The model under review builds one solid part; all positions refer to its coordinate system, in mm. A direction names the side the tool comes from. Coordinates: 2 decimals unless noted, no trailing zeros. Order: outer loops, then holes, each group sorted by start corner. A loop starts at its lowest first (then second) coordinate and runs counter-clockwise, first axis right, second up.
from build123d import *

# Parameters (mm, degrees)
SKETCH2_W                      = 17
SKETCH2_H                      = 17
BOSS_EXTRUDE1_DEPTH            = 3
SKETCH3_R                      = 2.2
CUT_EXTRUDE1_DEPTH             = 1.5
M2_CLEARANCE_HOLE1_D           = 2.4
M2_CLEARANCE_HOLE1_CSINK_D     = 2.45
M2_CLEARANCE_HOLE1_CSINK_ANGLE = 90
BOSS_EXTRUDE2_DEPTH            = 50
BOSS_EXTRUDE2_DRAFT            = 1.8
BOSS_EXTRUDE2_PROFILE_2_DEPTH  = 50
BOSS_EXTRUDE2_PROFILE_2_DRAFT  = 1.8
BOSS_EXTRUDE2_PROFILE_3_DEPTH  = 50
BOSS_EXTRUDE2_PROFILE_3_DRAFT  = 1.8
BOSS_EXTRUDE2_PROFILE_4_DEPTH  = 50
BOSS_EXTRUDE2_PROFILE_4_DRAFT  = 1.8
FILLET1_R                      = 6
FILLET2_R                      = 2
BOSS_EXTRUDE3_DEPTH            = 1.5


with BuildPart() as part:
    # Sketch2 → Boss-Extrude1 (new body)
    with BuildSketch(Plane(origin=(0, 0, 0), x_dir=(0, 1, 0), z_dir=(0, 0, 1))):
        with BuildLine():
            Line((-38.870057685, 34.627416998), (-34.627416998, 38.870057685))
            Line((-34.627416998, 38.870057685), (-14.186291501, 18.428932188))
            ThreePointArc((-14.186291501, 18.428932188), (-10.942058013, 16.261204675), (-7.115223689, 15.5))
            Line((-7.115223689, 15.5), (7.115223689, 15.5))
            ThreePointArc((7.115223689, 15.5), (10.942058013, 16.261204675), (14.186291501, 18.428932188))
            Line((14.186291501, 18.428932188), (34.627416998, 38.870057685))
            Line((34.627416998, 38.870057685), (38.870057685, 34.627416998))
            Line((38.870057685, 34.627416998), (18.428932188, 14.186291501))
            ThreePointArc((18.428932188, 14.186291501), (16.261204675, 10.942058013), (15.5, 7.115223689))
            Line((15.5, 7.115223689), (15.5, -7.115223689))
            ThreePointArc((15.5, -7.115223689), (16.261204675, -10.942058013), (18.428932188, -14.186291501))
            Line((18.428932188, -14.186291501), (38.870057685, -34.627416998))
            Line((38.870057685, -34.627416998), (34.627416998, -38.870057685))
            Line((34.627416998, -38.870057685), (14.186291501, -18.428932188))
            ThreePointArc((14.186291501, -18.428932188), (10.942058013, -16.261204675), (7.115223689, -15.5))
            Line((7.115223689, -15.5), (-7.115223689, -15.5))
            ThreePointArc((-7.115223689, -15.5), (-10.942058013, -16.261204675), (-14.186291501, -18.428932188))
            Line((-14.186291501, -18.428932188), (-34.627416998, -38.870057685))
            Line((-34.627416998, -38.870057685), (-38.870057685, -34.627416998))
            Line((-38.870057685, -34.627416998), (-18.428932188, -14.186291501))
            ThreePointArc((-18.428932188, -14.186291501), (-16.261204675, -10.942058013), (-15.5, -7.115223689))
            Line((-15.5, -7.115223689), (-15.5, 7.115223689))
            ThreePointArc((-15.5, 7.115223689), (-16.261204675, 10.942058013), (-18.428932188, 14.186291501))
            Line((-18.428932188, 14.186291501), (-38.870057685, 34.627416998))
        make_face()
        Rectangle(SKETCH2_W, SKETCH2_H, mode=Mode.SUBTRACT)
    extrude(amount=BOSS_EXTRUDE1_DEPTH)

    # Sketch3 → Cut-Extrude1 (cut)
    with BuildSketch(Plane.XY.offset(3)):
        with Locations((-12.5, 12.5)):
            Circle(SKETCH3_R)
        with Locations((12.5, 12.5)):
            Circle(SKETCH3_R)
        with Locations((12.5, -12.5)):
            Circle(SKETCH3_R)
        with Locations((-12.5, -12.5)):
            Circle(SKETCH3_R)
    extrude(amount=-CUT_EXTRUDE1_DEPTH, mode=Mode.SUBTRACT)

    # M2 Clearance Hole1 (through all)
    with Locations(Plane.XY.offset(3)):
        with Locations((12.5, 12.5), (-12.5, -12.5), (-12.5, 12.5), (12.5, -12.5)):
            CounterSinkHole(M2_CLEARANCE_HOLE1_D / 2, M2_CLEARANCE_HOLE1_CSINK_D / 2, counter_sink_angle=M2_CLEARANCE_HOLE1_CSINK_ANGLE)


with BuildPart() as boss_extrude2_tool:
    # Sketch7 → Boss-Extrude2 (with draft: the straight prism first)
    with BuildSketch(Plane(origin=(0, 0, 0), x_dir=(1, 0, 0), z_dir=(0, 0, -1))):
        Polygon((28.263455967, 31.091883092), (31.091883092, 28.263455967), (38.162950904, 35.334523779), (35.334523779, 38.162950904), align=None)
    extrude(amount=BOSS_EXTRUDE2_DEPTH)
    # Boss-Extrude2: the draft: its side faces are tilted about the plane it starts from
    boss_extrude2_sides = [boss_extrude2_tool.faces().sort_by_distance(p)[0] for p in [
        (29.67766953, -29.67766953, -25),
        (34.627416998, -31.798989873, -25),
        (36.748737342, -36.748737342, -25),
        (31.798989873, -34.627416998, -25),
    ]]
    draft(boss_extrude2_sides, Plane(origin=(0, 0, 0), x_dir=(1, 0, 0), z_dir=(0, 0, -1)), BOSS_EXTRUDE2_DRAFT)


with BuildPart() as part_1:
    add(part.part)

    # Boss-Extrude2: add boss_extrude2_tool
    add(boss_extrude2_tool.part)


with BuildPart() as boss_extrude2_profile_2_tool:
    # Sketch7 → Boss-Extrude2 profile 2 (with draft: the straight prism first)
    with BuildSketch(Plane(origin=(0, 0, 0), x_dir=(1, 0, 0), z_dir=(0, 0, -1))):
        Polygon((31.091883092, -28.263455967), (28.263455967, -31.091883092), (35.334523779, -38.162950904), (38.162950904, -35.334523779), align=None)
    extrude(amount=BOSS_EXTRUDE2_PROFILE_2_DEPTH)
    # Boss-Extrude2 profile 2: the draft: its side faces are tilted about the plane it starts from
    boss_extrude2_profile_2_sides = [boss_extrude2_profile_2_tool.faces().sort_by_distance(p)[0] for p in [
        (29.67766953, 29.67766953, -25),
        (31.798989873, 34.627416998, -25),
        (36.748737342, 36.748737342, -25),
        (34.627416998, 31.798989873, -25),
    ]]
    draft(boss_extrude2_profile_2_sides, Plane(origin=(0, 0, 0), x_dir=(1, 0, 0), z_dir=(0, 0, -1)), BOSS_EXTRUDE2_PROFILE_2_DRAFT)


with BuildPart() as part_2:
    add(part_1.part)

    # Boss-Extrude2 profile 2: add boss_extrude2_profile_2_tool
    add(boss_extrude2_profile_2_tool.part)


with BuildPart() as boss_extrude2_profile_3_tool:
    # Sketch7 → Boss-Extrude2 profile 3 (with draft: the straight prism first)
    with BuildSketch(Plane(origin=(0, 0, 0), x_dir=(1, 0, 0), z_dir=(0, 0, -1))):
        Polygon((-28.263455967, -31.091883092), (-31.091883092, -28.263455967), (-38.162950904, -35.334523779), (-35.334523779, -38.162950904), align=None)
    extrude(amount=BOSS_EXTRUDE2_PROFILE_3_DEPTH)
    # Boss-Extrude2 profile 3: the draft: its side faces are tilted about the plane it starts from
    boss_extrude2_profile_3_sides = [boss_extrude2_profile_3_tool.faces().sort_by_distance(p)[0] for p in [
        (-29.67766953, 29.67766953, -25),
        (-34.627416998, 31.798989873, -25),
        (-36.748737342, 36.748737342, -25),
        (-31.798989873, 34.627416998, -25),
    ]]
    draft(boss_extrude2_profile_3_sides, Plane(origin=(0, 0, 0), x_dir=(1, 0, 0), z_dir=(0, 0, -1)), BOSS_EXTRUDE2_PROFILE_3_DRAFT)


with BuildPart() as part_3:
    add(part_2.part)

    # Boss-Extrude2 profile 3: add boss_extrude2_profile_3_tool
    add(boss_extrude2_profile_3_tool.part)


with BuildPart() as boss_extrude2_profile_4_tool:
    # Sketch7 → Boss-Extrude2 profile 4 (with draft: the straight prism first)
    with BuildSketch(Plane(origin=(0, 0, 0), x_dir=(1, 0, 0), z_dir=(0, 0, -1))):
        Polygon((-31.091883092, 28.263455967), (-28.263455967, 31.091883092), (-35.334523779, 38.162950904), (-38.162950904, 35.334523779), align=None)
    extrude(amount=BOSS_EXTRUDE2_PROFILE_4_DEPTH)
    # Boss-Extrude2 profile 4: the draft: its side faces are tilted about the plane it starts from
    boss_extrude2_profile_4_sides = [boss_extrude2_profile_4_tool.faces().sort_by_distance(p)[0] for p in [
        (-29.67766953, -29.67766953, -25),
        (-31.798989873, -34.627416998, -25),
        (-36.748737342, -36.748737342, -25),
        (-34.627416998, -31.798989873, -25),
    ]]
    draft(boss_extrude2_profile_4_sides, Plane(origin=(0, 0, 0), x_dir=(1, 0, 0), z_dir=(0, 0, -1)), BOSS_EXTRUDE2_PROFILE_4_DRAFT)


with BuildPart() as part_4:
    add(part_3.part)

    # Boss-Extrude2 profile 4: add boss_extrude2_profile_4_tool
    add(boss_extrude2_profile_4_tool.part)

    # Fillet1
    fillet1_edges = [part_4.edges().sort_by_distance(p)[0] for p in [
        (-29.67766953, -29.67766953, 0),
        (-29.67766953, 29.67766953, 0),
        (29.67766953, 29.67766953, 0),
        (29.67766953, -29.67766953, 0),
    ]]
    fillet(fillet1_edges, radius=FILLET1_R)

    # Fillet2
    # the kernel refuses this fillet: 2 mm, written as the material it takes off along each edge
    with BuildSketch(Plane(origin=(34.627416998, 38.870057685, -12), x_dir=(0.7071067811865476, -0.7071067811865476, 0), z_dir=(0, 0, 1)), Plane(origin=(38.870057685, 34.627416998, -12), x_dir=(-0.7071067811865476, -0.7071067811865476, 0), z_dir=(0, 0, 1)), Plane(origin=(38.870057685, -34.627416998, -12), x_dir=(-0.7071067811865476, -0.7071067811865476, 0), z_dir=(0, 0, 1)), Plane(origin=(34.627416998, -38.870057685, -12), x_dir=(-0.7071067811865476, 0.7071067811865476, 0), z_dir=(0, 0, 1)), Plane(origin=(-38.870057685, -34.627416998, -12), x_dir=(0.7071067811865476, 0.7071067811865476, 0), z_dir=(0, 0, 1)), Plane(origin=(-38.870057685, 34.627416998, -12), x_dir=(0.7071067811865476, 0.7071067811865476, 0), z_dir=(0, 0, 1)), Plane(origin=(-34.627416998, 38.870057685, -12), x_dir=(0.7071067811865476, -0.7071067811865476, 0), z_dir=(0, 0, 1))) as fillet2_piece_1:
        with BuildLine():
            CenterArc((FILLET2_R, -FILLET2_R), FILLET2_R, 90, 90)
            Line((0, -FILLET2_R), (-FILLET2_R * 0.02, -FILLET2_R))
            Line((-FILLET2_R * 0.02, -FILLET2_R), (-FILLET2_R * 0.02, FILLET2_R * 0.02))
            Line((-FILLET2_R * 0.02, FILLET2_R * 0.02), (FILLET2_R, FILLET2_R * 0.02))
            Line((FILLET2_R, FILLET2_R * 0.02), (FILLET2_R, 0))
        make_face()
    extrude(amount=27, mode=Mode.SUBTRACT)
    with BuildSketch(Plane(origin=(-34.627416998, -38.870057685, -12), x_dir=(0.7071067811865458, 0.7071067811865493, 0), z_dir=(0, 0, 1))) as fillet2_piece_2:
        with BuildLine():
            CenterArc((FILLET2_R, FILLET2_R), FILLET2_R, 180, 90)
            Line((0, FILLET2_R), (-FILLET2_R * 0.02, FILLET2_R))
            Line((-FILLET2_R * 0.02, FILLET2_R), (-FILLET2_R * 0.02, -FILLET2_R * 0.02))
            Line((-FILLET2_R * 0.02, -FILLET2_R * 0.02), (FILLET2_R, -FILLET2_R * 0.02))
            Line((FILLET2_R, -FILLET2_R * 0.02), (FILLET2_R, 0))
        make_face()
    extrude(amount=27, mode=Mode.SUBTRACT)

    # Sketch8 → Boss-Extrude3 (add)
    with BuildSketch(Plane.XY.offset(3)):
        Polygon((-16.207106781, 14.792893219), (-14.792893219, 16.207106781), (-33.17766953, 34.591883092), (-34.591883092, 33.17766953), align=None)
        Polygon((14.792893219, 16.207106781), (16.207106781, 14.792893219), (34.591883092, 33.17766953), (33.17766953, 34.591883092), align=None)
        Polygon((16.207106781, -14.792893219), (14.792893219, -16.207106781), (33.17766953, -34.591883092), (34.591883092, -33.17766953), align=None)
        Polygon((-14.792893219, -16.207106781), (-16.207106781, -14.792893219), (-34.591883092, -33.17766953), (-33.17766953, -34.591883092), align=None)
    extrude(amount=BOSS_EXTRUDE3_DEPTH)


solid = part_4.part
(1) Consider section A-A (x = -12.5). Give the boundary of the cut face in (y, z).
(2) The part is to be moulded in two halves that separate along Y. For faces 1 (the face through (0, 15.5, 1)), 2 (the face through (25.271, 23.857, 3.74)), 3 (the face through (-10.89, -16.24, 1.48)), say which applies: +Y half, -Y half, draft (parallel to the pull), parting line (faces both ways), or undercut.
(3) Tool access review of faces 4 (the face through (-9, 0, 3)), 5 (the face through (-8.5, 0, 1)), 6 (the face through (23.833, -28.076, 1.479)): name each direction out of +Z, -Z, +X, -X, +Y, -Y from which nothing blocks a thin tool from reaching the whole face with its end or side.
(4) Consider section D-D (y = -20.5). Give the boundary of the cut face in (x, z), then the cut area to 3 significant figures.
(5) Consider section C-C (z = -37). Give the boundary of the cut face in (x, y).
(6) Insertion check: pin 1 Ø1.5 at (x, z) = (4, 2) entering from +Y; pin 2 Ø3.5 at (x, y) = (-12, 13.5) entering from +Z; pin 3 Ø4 at (x, y) = (-12.5, -12.5) entering from +Z. Each pin has a flat end and moves straight along its axis. Give the tip position at first contact, or say it passes through.
(7) Wall thickness on line 1 (X direction, y = 14, z = 2.5); line 2 (X direction, y = 7.5, z = 1.5); line 3 (Y direction, x = 12.5, z = 0.75): over which ranges is each line inside the solid? List them lowest first.
(8) Consider section B-B (x = -21.5). Give the boundary of the cut face in (y, z), then the cut area to 3 significant figures.
Findings:
1. outline: (-17.07, 0) - (-13.7, 0) - (-13.7, 1.5) - (-14.7, 1.5) - (-14.7, 3) - (-17.07, 3) - close; (-11.3, 0) - (11.3, 0) - (11.3, 1.5) - (10.3, 1.5) - (10.3, 3) - (-10.3, 3) - (-10.3, 1.5) - (-11.3, 1.5) - close; (13.7, 0) - (17.07, 0) - (17.07, 3) - (14.7, 3) - (14.7, 1.5) - (13.7, 1.5) - close
2. face 1: +Y half
2. face 2: undercut
2. face 3: -Y half
3. face 4: +Z
3. face 5: +Z, -Z
3. face 6: +Z, -Z, -Y
4. outline: (-24.74, 0) - (-16.26, 0) - (-16.26, 3) - (-19.09, 3) - (-19.09, 4.5) - (-21.91, 4.5) - (-21.91, 3) - (-24.74, 3) - close; (16.26, 0) - (24.74, 0) - (24.74, 3) - (21.91, 3) - (21.91, 4.5) - (19.09, 4.5) - (19.09, 3) - (16.26, 3) - close
4. area: 59.4 mm2
5. outline: (-36.52, -35.33) - (-35.33, -36.52) - (-29.91, -31.09) - (-31.09, -29.91) - close; (-36.52, 35.33) - (-31.09, 29.91) - (-29.91, 31.09) - (-35.33, 36.52) - close; (29.91, -31.09) - (35.33, -36.52) - (36.52, -35.33) - (31.09, -29.91) - close; (29.91, 31.09) - (31.09, 29.91) - (36.52, 35.33) - (35.33, 36.52) - close
6. pin 1: stops at y = 15.5
6. pin 2: stops at z = 3
6. pin 3: stops at z = 1.5
7. line 1: x = -18.25 to -14.11, -10.89 to 10.89, 14.11 to 18.25
7. line 2: x = -15.51 to -8.5, 8.5 to 15.51
7. line 3: y = -17.07 to -13.7, -11.3 to 11.3, 13.7 to 17.07
8. outline: (-25.74, 0) - (-17.26, 0) - (-17.26, 3) - (-20.09, 3) - (-20.09, 4.5) - (-22.91, 4.5) - (-22.91, 3) - (-25.74, 3) - close; (17.26, 0) - (25.74, 0) - (25.74, 3) - (22.91, 3) - (22.91, 4.5) - (20.09, 4.5) - (20.09, 3) - (17.26, 3) - close
8. area: 59.4 mm2
